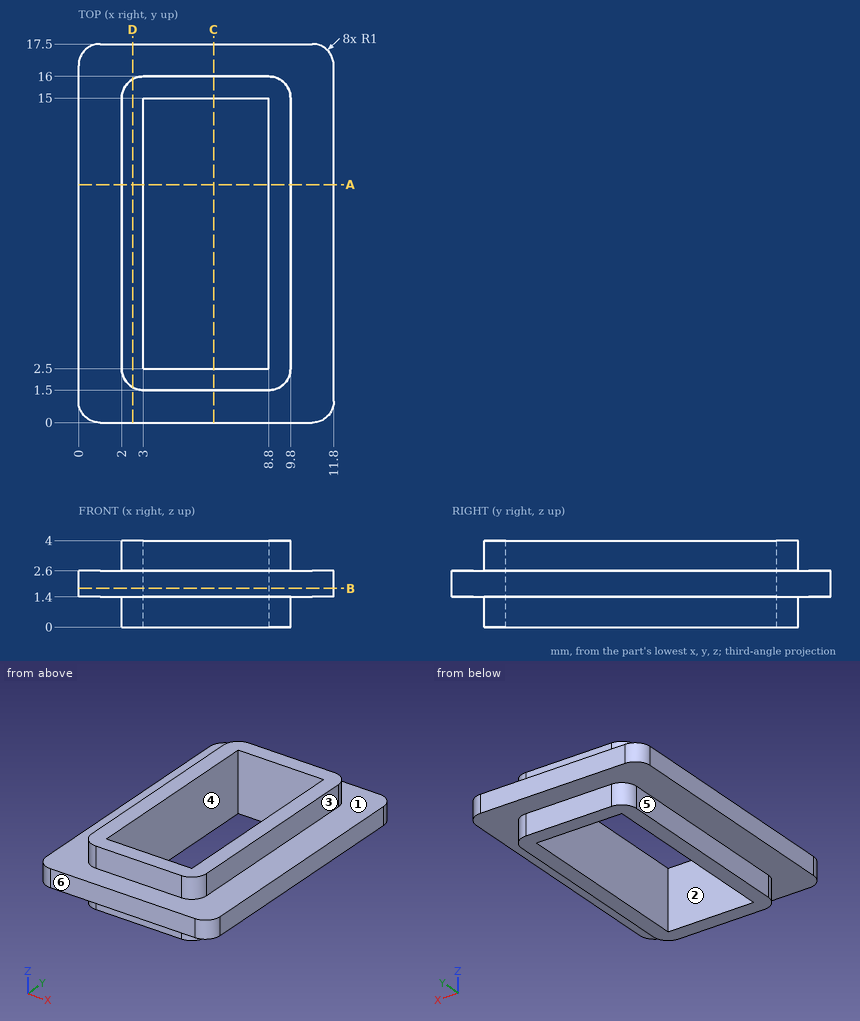
Study the drawing (mm; zero at the part's minimum x, y, z) and answer. A direction names the side the tool comes from. Give positions to 0.01 mm unless a question says otherwise; leave off trailing zeros. Order: outer loops, then holes, each group sorted by start corner. A loop starts at its lowest first (then second) coordinate and runs counter-clockwise, first axis right, second up. Notation, with made-up numbers: M 77.25,15 L 133.25,15 A36 cw 133.25,49 Z; hole C 85,70.25 d11. An arc over 180 degrees is marked long. Put each result on its own line as item: value. Start each with the question number.
Item 1: The part is cut by section A-A, the plane y = 11. Determine the outline of the cut face in (x, z), and give its area (3 significant figures).
Item 2: Flat-ended cylindrical pins translate along their axes: P1, Ø1.5, axis at x = 2.5, z = 1, coming from the +Y side; P2, Ø0.7, axis at x = 6.5, z = 1, coming from the +Y side; P3, Ø2, axis at x = 5.5, y = 7.5, coming from the -Z side. Find the tip coordinate at first contact, or state that the pin passes through.
Item 3: The part is cut by section C-C, the plane x = 6.25. Determine the outline of the cut face in (y, z).
Item 4: Find the intervals of material crossed by line 1 along X through (y, z) = (14.5, 1); line 2 along X through (y, z) = (8, 1.7); line 3 along Y through (x, z) = (8.75, 2.8), in increasing order.
Item 5: For a pull along X with two mould halves and no side action, classify the marked faces 4, 5 and 6 as +X half, -X half, draft (parallel to the pull), parting line (faces both ways), or undercut.
Item 6: Which of the six approach directions +Z, -Z, +X, -X, +Y, -Y give full straight-line access (tool end or side, diameter ignored) to the marked faces 1, 2 and 3?
Item 7: The part is cut by section B-B, the plane z = 1.8. Determine the outline of the cut face in (x, y), and give its area (3 significant figures).
Item 8: The part is cut by section D-D, the plane x = 2.5. Determine the outline of the cut face in (y, z), and give its area (3 significant figures).
Answer key:
1. outline: M 0,1.4 L 2,1.4 L 2,0 L 3,0 L 3,4 L 2,4 L 2,2.6 L 0,2.6 Z; M 8.8,0 L 9.8,0 L 9.8,1.4 L 11.8,1.4 L 11.8,2.6 L 9.8,2.6 L 9.8,4 L 8.8,4 Z
1. area: 12.8 mm²
2. P1: stops at y = 17.5
2. P2: stops at y = 16
2. P3: passes through
3. outline: M 0,1.4 L 1.5,1.4 L 1.5,0 L 2.5,0 L 2.5,4 L 1.5,4 L 1.5,2.6 L 0,2.6 Z; M 15,0 L 16,0 L 16,1.4 L 17.5,1.4 L 17.5,2.6 L 16,2.6 L 16,4 L 15,4 Z
4. line 1: x = 2 to 3, 8.8 to 9.8
4. line 2: x = 0 to 3, 8.8 to 11.8
4. line 3: y = 1.5 to 2.5, 15 to 16
5. face 4: undercut
5. face 5: -X half
5. face 6: draft
6. face 1: +Z
6. face 2: +Z, -Z
6. face 3: +Z, +X, +Y, -Y
7. outline: M 0,1 A1 ccw 1,0 L 10.8,0 A1 ccw 11.8,1 L 11.8,16.5 A1 ccw 10.8,17.5 L 1,17.5 A1 ccw 0,16.5 Z; hole M 3,2.5 L 8.8,2.5 L 8.8,15 L 3,15 Z
7. area: 133 mm²
8. outline: M 0,1.4 L 1.63,1.4 L 1.63,0 L 15.87,0 L 15.87,1.4 L 17.5,1.4 L 17.5,2.6 L 15.87,2.6 L 15.87,4 L 1.63,4 L 1.63,2.6 L 0,2.6 Z
8. area: 60.8 mm²
